Answer from the drawing. Dimensions are ordinates in mm from the lowest x, y and z of the part. Round coordinates to 2 decimals unless told otherwise and drop trailing zeros. Write each loop counter-clockwise with the first axis right and the second up, starting at its lowest first coordinate (ties: lowest second). Pieces come first, ordered by that corner, then holes. Notation, with made-up numbers: M 57,64.25 L 100,64.25 A23 ccw 100,92.25 Z; hole C 43.5,46.25 d9. An arc over 180 degrees is marked long. One line per item, written item: value. Start each with the question number.
(1) Section A-A (z = 16.5) is taken. Determine the outline of the cut face in (x, y).
(2) Section C-C (x = 18.5) is taken. Determine the outline of the cut face in (y, z).
(3) Consider probe 1 along Z at (x, y) = (21.5, 0.95); probe 2 along Z at (x, y) = (4.5, 1.85); probe 3 along X at (y, z) = (1.2, 25). Determine where each line is inside the solid, lowest interval first.
(4) Given P1, Ø3, axis at x = 23.9, z = 36.8, coming from the -Y side; P2, Ø1, axis at x = 32, y = 1.5, coming from the +Z side; P3, Ø1.5, axis at y = 1.5, z = 35, coming from the -X side; P4, Ø1.5, axis at y = 1, z = 22, coming from the +X side, each flat-ended and moving along its own axis, determine where each tip first touches the part or whether it passes through.
(5) Section B-B (y = 1.1) is taken. Determine the outline of the cut face in (x, z) (3 decimals), plus the area to 3 significant figures.
(6) Section D-D (z = 10.5) is taken. Determine the outline of the cut face in (x, y), plus the area to 3 significant figures.
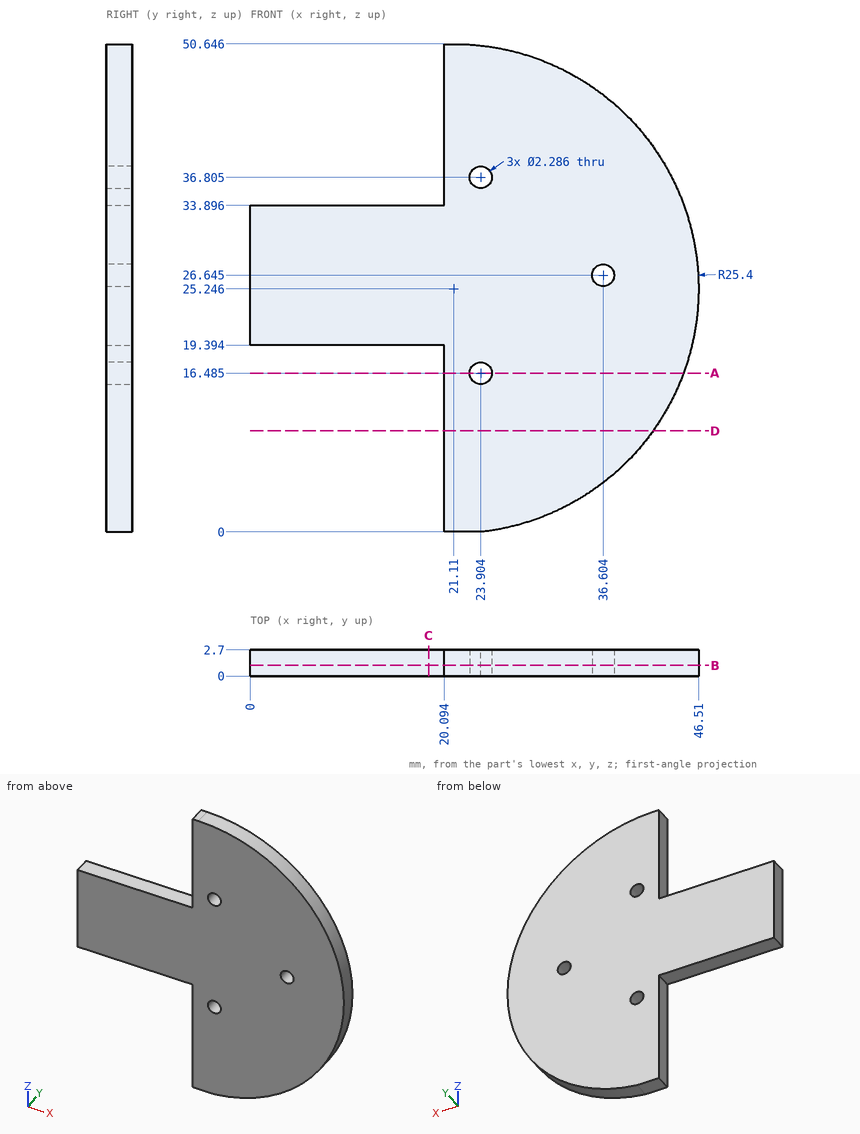
Recorded:
1. outline: M 20.09,0 L 22.76,0 L 22.76,2.7 L 20.09,2.7 Z; M 25.05,0 L 44.96,0 L 44.96,2.7 L 25.05,2.7 Z
2. outline: M 0,19.39 L 2.7,19.39 L 2.7,33.9 L 0,33.9 Z
3. probe 1: z = 0 to 50.64
3. probe 2: z = 19.39 to 33.9
3. probe 3: x = 0 to 46.51
4. P1: stops at y = 0
4. P2: stops at z = 48.42
4. P3: stops at x = 20.09
4. P4: stops at x = 46.39
5. outline: M 0,19.394 L 20.094,19.394 L 20.094,0 L 23.904,0 A25.4 ccw 21.11,50.646 L 20.094,50.646 L 20.094,33.896 L 0,33.896 Z; hole C 23.904,16.485 d2.286; hole C 23.904,36.805 d2.286; hole C 36.604,26.645 d2.286
5. area: 1,340 mm2
6. outline: M 20.09,0 L 41.79,0 L 41.79,2.7 L 20.09,2.7 Z
6. area: 58.6 mm2
